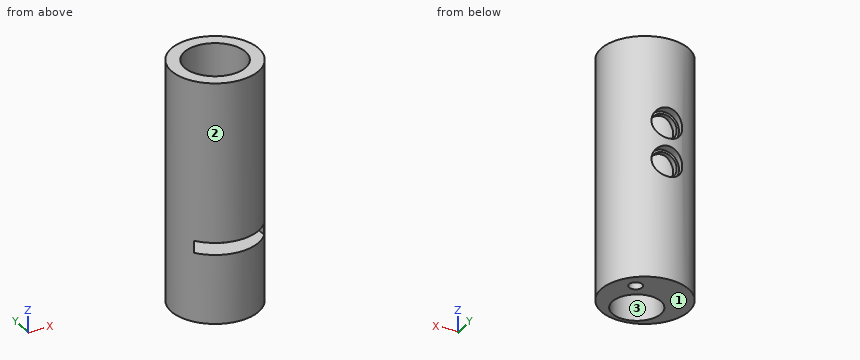
Autodesk Inventor part; units mm, degrees
ref_plane "Work Plane2" through (0, 20, 0) normal (0, 1, 0) x (-1, 0, 0)
ref_plane "Work Plane5" through (0, 13, 71.5) normal (0, 1, 0) x (1, 0, 0)
ref_plane "YZ Plane" through (0, 0, 0) normal (1, 0, 0) x (0, 1, 0)
sketch "Sketch1" plane through (0, 0, 0) normal (0, 0, 1) x (1, 0, 0)
  circle A0 centre (0, 0) radius 20
  dimension "d0" = 40
extrude "Extrusion1" add sketch "Sketch1" along normal blind 110
ref_plane "Work Plane2" through (0, 20, 0) normal (0, 1, 0) x (-1, 0, 0)
sketch "Sketch3" plane through (0, 20, 0) normal (0, 1, 0) x (-1, 0, 0)
  circle A0 centre (0, 54) radius 7
  circle A1 centre (0, 71.5) radius 7
  point P0 (0, 0)
  dimension "d3" = 14
  dimension "d4" = 14
  dimension "d5" = 17.5
  dimension "d6" = 54
  dimension "d7" = 0
  dimension "d8" = 0
extrude "Extrusion2" cut sketch "Sketch3" against normal blind 4
sketch "Sketch4" plane through (0, 16, 71.5) normal (0, 1, 0) x (1, 0, 0)
  circle A0 centre (0, 0) radius 7
  circle A1 centre (0, 0) radius 5.9531
  circle A2 centre (0, 17.5) radius 7
  circle A3 centre (0, 17.5) radius 5.9531
  point P0 (0, 71.5)
  dimension "d11" = 11.9062
  dimension "d12" = 11.9062
extrude "Extrusion3" cut sketch "Sketch4" against normal blind 23 contours A1 | A3
sketch "Sketch5" plane through (0, 0, 0) normal (0, 0, -1) x (-1, 0, 0)
  circle A0 centre (0, -7) radius 11.125
  point P0 (0, 0)
  dimension "d15" = 22.25
  dimension "d40" = 0
  dimension "d63" = 7
extrude "Extrusion4" cut sketch "Sketch5" against normal blind 15
sketch "Sketch6" plane through (0, -7, 15) normal (0, 0, -1) x (-1, 0, 0)
  circle A0 centre (0, 0) radius 5.85
  circle A1 centre (0, 0) radius 11.125
  point P0 (0, 7)
  dimension "d19" = 11.7
extrude "Extrusion5" cut sketch "Sketch6" against normal blind 0.3 contours A0
sketch "Sketch7" plane through (0, -7, 15.3) normal (0, 0, -1) x (-1, 0, 0)
  circle A0 centre (0, 0) radius 5
  circle A1 centre (0, 0) radius 5.85
  point P0 (0, 7)
  dimension "d22" = 10
extrude "Extrusion6" cut sketch "Sketch7" against normal blind 9 contours A0
sketch "Sketch8" plane through (0, -7, 24.3) normal (0, 0, -1) x (-1, 0, 0)
  circle A0 centre (0, 0) radius 3.5
  circle A1 centre (0, 0) radius 5
  point P0 (0, 7)
  dimension "d25" = 7
extrude "Extrusion7" cut sketch "Sketch8" against normal blind 18 contours A0
sketch "Sketch9" plane through (0, -7, 15) normal (0, 0, -1) x (-1, 0, 0)
  circle A0 centre (-7.4, 0) radius 1.25
  circle A1 centre (0, 0) radius 3.5
  point P0 (0, 7)
  dimension "d28" = 2.5
  dimension "d29" = 7.4
  dimension "d30" = 0
extrude "Extrusion8" cut sketch "Sketch9" against normal blind 2 contours A0
ref_plane "Work Plane3" through (0, -7, 34.3) normal (0, 0, -1) x (-1, 0, 0)
sketch "Sketch11" plane through (0, -7, 34.3) normal (0, 0, -1) x (-1, 0, 0)
  circle A0 centre (0, 0) radius 3.5
  arc A1 (16, 0) -> (-16, 0) centre (0, 0) ccw
  line L0 (16, 0) -> (16, -16)
  line L1 (16, -16) -> (-16, -16)
  line L2 (-16, -16) -> (-16, 0)
  point P0 (0, 7)
  dimension "d37" = 32
extrude "Extrusion10" cut sketch "Sketch11" along normal mid plane 5.5
sketch "Sketch12" plane through (0, 0, 0) normal (0, 0, -1) x (-1, 0, 0)
  circle A0 centre (-9, 9) radius 3
  circle A1 centre (0, 0) radius 20
  dimension "d58" = 6
  dimension "d59" = 9
  dimension "d60" = 9
sketch "Sketch13" plane through (0, 0, 110) normal (0, 0, 1) x (1, 0, 0)
  circle A0 centre (0, 0) radius 14
  dimension "d44" = 28
extrude "Extrusion11" cut sketch "Sketch13" against normal blind 65
ref_plane "Work Plane5" through (0, 13, 71.5) normal (0, 1, 0) x (1, 0, 0)
sketch "Sketch15" plane through (0, 13, 71.5) normal (0, 1, 0) x (1, 0, 0)
  circle A0 centre (0, 17.5) radius 7
  circle A1 centre (0, 17.5) radius 8.5
  circle A2 centre (0, 0) radius 7
  circle A3 centre (0, 0) radius 8.5
  point P0 (0, 71.5)
  dimension "d54" = 17
  dimension "d55" = 17
extrude "Extrusion14" cut sketch "Sketch15" against normal blind 10 contours A0 | A2
extrude "Extrusion15" cut sketch "Sketch12" against normal up to surface (45 mm away) contours A0
properties part number "Housing"
CAD build for the part. Positions are in the model's coordinates, mm. Face numbers are marked on the shaded views. Round coordinates to 2 decimals unless told otherwise and drop trailing zeros. Write each loop counter-clockwise with the first axis right and the second up, starting at its lowest first coordinate (ties: lowest second). Pieces come first, ordered by that corner, then holes.
(1) Slice it at A-A, the plane y = 1.5. Write the cut outline in (x, z), and give its area (3 significant figures).
(2) Slice it at C-C, the plane x = 15. Write the cut outline in (y, z), and give its area (3 significant figures).
(3) Mould opens along Y. For the marked faces 1, 2 and 3 say: pulls with the +Y half, pulls with the -Y half, needs draft (parallel to the pull), parting line crosses it, or undercut.
(4) Drop flat-ended pins along their axis: P1, Ø13.5, axis at x = 0, z = 71.5, coming from the +Y side; P2, Ø3, axis at x = 7.4, y = -7, coming from the -Z side; P3, Ø6, axis at x = -3, z = 38.5, coming from the -Y side; P4, Ø1, axis at x = -15, z = 83.5, coming from the -Y side (3 decimals). Give the stop position or say it passes through.
(5) Slice it at D-D, the plane z = 71.5. Write the cut outline in (x, y) (3 decimals).
(6) Probe line 1 along Z through (x, y) = (-11, -11.5); line 2 along Y through (x, z) = (0, 8.75) (3 decimals); line 3 along Z through (x, y) = (11, -3). List the from-to ranges inside material, lowest first.
(7) Slice it at B-B, the plane z = 23. Write the cut outline in (x, y), and give its area (3 significant figures).
From the geometry:
1. outline: (-19.94, 0) - (-7.18, 0) - (-7.18, 15) - (7.18, 15) - (7.18, 0) - (19.94, 0) - (19.94, 110) - (13.92, 110) - (13.92, 45) - (-13.92, 45) - (-13.92, 110) - (-19.94, 110) - close; hole (-13.56, 31.55) - (13.56, 31.55) - (13.56, 37.05) - (-13.56, 37.05) - close
1. area: 2,210 mm2
2. outline: (-13.23, 0) - (13.23, 0) - (13.23, 110) - (-13.23, 110) - (-13.23, 37.05) - (-1.43, 37.05) - (-1.43, 31.55) - (-13.23, 31.55) - close
2. area: 2,850 mm2
3. face 1: needs draft
3. face 2: parting line crosses it
3. face 3: undercut
4. P1: stops at y = 16
4. P2: stops at z = 15
4. P3: stops at y = -20
4. P4: stops at y = -13.775
5. outline: (-7, 12.124) - (-7, 13) - (-5.953, 13) - (-5.953, 16) - (-7, 16) - (-7, 18.735) arc R20 ccw (long way) to (7, 18.735) - (7, 16) - (5.953, 16) - (5.953, 13) - (7, 13) - (7, 12.124) arc R14 cw (long way) to start
6. line 1: z = 0 to 31.55, 37.05 to 110
6. line 2: y = -20 to -18.125, 4.125 to 20
6. line 3: z = 0 to 31.55, 37.05 to 45
7. outline: circle Ø40 at (0, 0); hole circle Ø10 at (0, -7); hole circle Ø6 at (9, 9)
7. area: 1,150 mm2
